Can you work these out from the model? Positions are in its coordinate system, mm. A direction names the side the tool comes from. Coordinates: 2 decimals unless noted, no trailing zeros. Loops run counter-clockwise (first coordinate to the right, second up) from the corner with the lowest first, then second, coordinate; pieces in that order, holes last.
```python
from build123d import *

# Parameters (mm, degrees)
BOSS_EXTRUDE1_DEPTH = 9.525
CUT_EXTRUDE1_REACH  = 84.186
SKETCH3_R           = 3.3782
FILLET1_R           = 3.175


with BuildPart() as part:
    # Sketch2 → Boss-Extrude1 (new, symmetric)
    with BuildSketch(Plane.XY):
        with BuildLine():
            Line((47.625, 0), (66.300169076, 0))
            Line((66.300169076, 0), (66.300169076, 6.35))
            Line((66.300169076, 6.35), (53.600169076, 6.35))
            ThreePointArc((53.600169076, 6.35), (0, 53.975), (-53.600169076, 6.35))
            Line((-53.600169076, 6.35), (-66.300169076, 6.35))
            Line((-66.300169076, 6.35), (-66.300169076, 0))
            Line((-66.300169076, 0), (-47.625, 0))
            ThreePointArc((-47.625, 0), (0, 47.625), (47.625, 0))
        make_face()
    extrude(amount=BOSS_EXTRUDE1_DEPTH, both=True)

    # Sketch3 → Cut-Extrude1 (cut, up to next)
    with BuildSketch(Plane(origin=(0, 6.35, 0), x_dir=(1, 0, 0), z_dir=(0, 1, 0)), mode=Mode.PRIVATE) as cut_extrude1_sk1:
        with Locations(Location((59.950169076, 0, 0), (0, 0, 180))):
            Circle(SKETCH3_R)
    cut_extrude1_tool1 = extrude(cut_extrude1_sk1.sketch, amount=-CUT_EXTRUDE1_REACH, mode=Mode.PRIVATE) & part.part
    # Sketch3 → Cut-Extrude1 (cut, up to next)
    with BuildSketch(Plane(origin=(0, 6.35, 0), x_dir=(1, 0, 0), z_dir=(0, 1, 0)), mode=Mode.PRIVATE) as cut_extrude1_sk2:
        with Locations(Location((-59.950169076, 0, 0), (0, 0, 270))):
            Circle(SKETCH3_R)
    cut_extrude1_tool2 = extrude(cut_extrude1_sk2.sketch, amount=-CUT_EXTRUDE1_REACH, mode=Mode.PRIVATE) & part.part
    add(cut_extrude1_tool1.solids().sort_by_distance((59.950169, 6.35, 0))[0], mode=Mode.SUBTRACT)
    add(cut_extrude1_tool2.solids().sort_by_distance((-59.950169, 6.35, 0))[0], mode=Mode.SUBTRACT)

    # Fillet1
    fillet1_edges = [part.edges().sort_by_distance(p)[0] for p in [
        (66.300169076, 3.175, -9.525),
        (66.300169076, 3.175, 9.525),
        (-47.625, 0, 0),
        (47.625, 0, 0),
        (-66.300169076, 3.175, 9.525),
        (-66.300169076, 3.175, -9.525),
    ]]
    fillet(fillet1_edges, radius=FILLET1_R)


solid = part.part
```
Item 1: Suppose I cut it at D-D, the plane x = 41. Please give me the cut outline in (y, z) (3 decimals).
Results are:
outline: (24.231, -9.525) - (35.104, -9.525) - (35.104, 9.525) - (24.231, 9.525) - close
Item 2: On a 3-axis mill with a long thin cutter (end or side, diameter ignored), from which of +Z, -Z, +X, -X, +Y, -Y can I reach the whole of each face in a straight line? I mean faces 4 (the face through (-57, 6.35, -2)), 5 (the face through (57, 6.35, 2)), 6 (the face through (48.55, 0.84, -0.13)), 7 (the face through (-65.345, 3.131, -8.62)), 8 (the face through (65.395, 3.219, 8.57)). Say none if no direction works.
Results are:
face 4: +Z, -Z, -X, +Y
face 5: +Z, -Z, +X, +Y
face 6: +Z, -Z, -Y
face 7: -Z, -X, +Y, -Y
face 8: +Z, +X, +Y, -Y
Item 3: We'd pull the mould along X, two halves only. Please class faces 1 (the face through (-1.006, 47.614, 0.133)), 2 (the face through (-57, 0, -2)), 3 (the face through (-66.3, 3, 0)): +X half, -X half, draft (parallel to the pull), parting line (faces both ways), or undercut.
Results are:
face 1: undercut
face 2: draft
face 3: -X half
Item 4: Suppose I cut it at B-B, the plane z = 0. Please give me the cut outline in (x, y) (3 decimals), plus the area to 3 significant figures.
Results are:
outline: (-66.3, 0) - (-63.328, 0) - (-63.328, 6.35) - (-66.3, 6.35) - close; (-56.572, 0) - (-50.701, 0) arc R3.175 ccw to (-47.532, 2.977) arc R47.625 cw to (47.532, 2.977) arc R3.175 ccw to (50.701, 0) - (56.572, 0) - (56.572, 6.35) - (53.6, 6.35) arc R53.975 ccw to (-53.6, 6.35) - (-56.572, 6.35) - close; (63.328, 0) - (66.3, 0) - (66.3, 6.35) - (63.328, 6.35) - close
area: 1,080 mm2
Item 5: I'm going to push flat-ended pins straight in: P1, Ø1.5, axis at x = 0, y = 45, coming from the +Z side; P2, Ø3, axis at x = 48, z = 0.5, coming from the -Y side; P3, Ø8, axis at x = 39, z = 5.5, coming from the -Y side; P4, Ø1, axis at x = 7.5, z = 6.5, coming from the +Y side. Where does each tip first touch, or does it pass through?
Results are:
P1: passes through
P2: stops at y = 0.24
P3: stops at y = 20.47
P4: stops at y = 53.52
Item 6: Suppose I cut it at C-C, the plane x = 4. Please give me the cut outline in (y, z) (3 decimals), plus the area to 3 significant figures.
Results are:
outline: (47.457, -9.525) - (53.827, -9.525) - (53.827, 9.525) - (47.457, 9.525) - close
area: 121 mm2
Item 7: I need wall thicknesses on line 1 along Y through (x, z) = (-58.5, -7.75); line 2 along X through (y, z) = (25.5, -4); line 3 along X through (y, z) = (21.5, -5.5). Which ranges of each line are inside material? Lowest first, please.
Results are:
line 1: y = 0 to 6.35
line 2: x = -47.57 to -40.22, 40.22 to 47.57
line 3: x = -49.51 to -42.5, 42.5 to 49.51
Item 8: Suppose I cut it at A-A, the plane y = 36. Please give me the cut outline in (x, z) (3 decimals).
Results are:
outline: (-40.216, -9.525) - (-31.179, -9.525) - (-31.179, 9.525) - (-40.216, 9.525) - close; (31.179, -9.525) - (40.216, -9.525) - (40.216, 9.525) - (31.179, 9.525) - close
